Source: CAD feature listing. Evaluate the final solid. Frame: model axes, mm. Face numbers are marked on the shaded views. A direction names the side the tool comes from. Coordinates: 2 decimals unless noted, no trailing zeros. Order: outer loops, then holes, each group sorted by start corner. A loop starts at its lowest first (then second) coordinate and runs counter-clockwise, first axis right, second up. Notation, with made-up numbers: (-2.75, 70) -> (3.25, 70) arc R22 ccw to (3.25, 79) -> close; hole circle Ø4 at (8, 63). An arc over 180 degrees is marked (long way). Put each result on its own line as item: value.
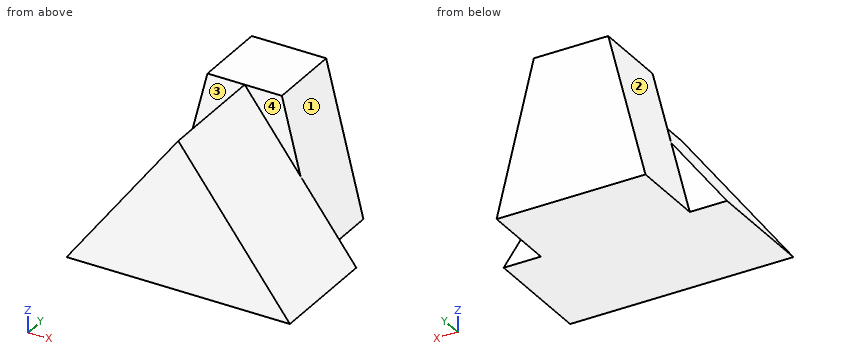
from build123d import *

# Parameters (mm, degrees)
BOSS_EXTRUDE1_DEPTH = 3
BOSS_EXTRUDE2_DEPTH = 2


with BuildPart() as part:
    # Sketch1 → Boss-Extrude1 (new body)
    with BuildSketch(Plane(origin=(0, 0, 0), x_dir=(1, 0, 0), z_dir=(0, 1, 0))):
        Polygon((0, 0), (-3, 4), (3, 4), align=None)
    extrude(amount=BOSS_EXTRUDE1_DEPTH)

    # Sketch2 → Boss-Extrude2 (add)
    with BuildSketch(Plane(origin=(0, 3, 0), x_dir=(1, 0, 0), z_dir=(0, 1, 0))):
        Polygon((2, 4), (1, 0), (-1, 0), (-2, 4), align=None)
    extrude(amount=BOSS_EXTRUDE2_DEPTH)


solid = part.part
1. Cut plane C-C on x = -1.65. Output: boundary loops of the cut face in (y, z), plus the area to 3 significant figures.
Numbers:
outline: (0, -4) -> (5, -4) -> (5, -2.6) -> (3, -2.6) -> (3, -2.2) -> (0, -2.2) -> close
area: 8.20 mm2
2. Cut plane B-B on z = -0.55. Output: boundary loops of the cut face in (x, y).
Numbers:
outline: (-1.14, 3) -> (-0.41, 3) -> (-0.41, 0) -> (0.41, 0) -> (0.41, 3) -> (1.14, 3) -> (1.14, 5) -> (-1.14, 5) -> close
3. Ray query, line 1 along Y through (x, z) = (-1.15, -1.4); line 2 along Z through (x, y) = (-1.5, 0.4); line 3 along X through (y, z) = (0.55, -0.5) (3 decimals). Return the intervals inside material, ascending.
Numbers:
line 1: y = 3 to 5
line 2: z = -4 to -2
line 3: x = -0.375 to 0.375
4. Cut plane D-D on y = 2.6. Output: boundary loops of the cut face in (x, z), plus the area to 3 significant figures.
Numbers:
outline: (-3, -4) -> (3, -4) -> (0, 0) -> close
area: 12.0 mm2
5. First-contact query: pin 1 (1 mm diameter, centred on y = 4, z = -1.5, fed in from -X); pin 2 (1.5 mm diameter, centred on y = 1, z = -2.5, fed in from -X); pin 3 (2 mm diameter, centred on y = 4, z = -1.5, fed in from +X) (3 decimals). Flat tips, straight axial feed; report the tip coordinate or a pass-through.
Numbers:
pin 1: stops at x = -1.5
pin 2: stops at x = -2.44
pin 3: stops at x = 1.625
6. Cut plane A-A on x = 1.2. Output: boundary loops of the cut face in (y, z).
Numbers:
outline: (0, -4) -> (5, -4) -> (5, -0.8) -> (3, -0.8) -> (3, -1.6) -> (0, -1.6) -> close
7. Set-up query: the marked faces 1, 2, 3 and 4. Return all of +Z, -Z, +X, -X, +Y, -Y with unobstructed straight access to the full face (end or side cutting, diameter ignored); none if empty.
Numbers:
face 1: +Z, +X, +Y
face 2: +Z, -X, +Y
face 3: +Z, -X, -Y
face 4: +Z, +X, -Y
